Geometry: final body of the model. Coordinates: model frame, mm. Coordinates: 2 decimals unless noted, no trailing zeros. Loops run counter-clockwise (first coordinate to the right, second up) from the corner with the lowest first, then second, coordinate; pieces in that order, holes last. Notation, with made-up numbers: (-33.75, 0.5) - (-9.75, 0.5) arc R27 cw to (-9.75, 32.5) - close; hole circle Ø7 at (-10.75, 64.5). An arc over 180 degrees is marked (long way). Return JSON: item names as keys, results as strings.
from build123d import *

# Parameters (mm, degrees)
F0_W     = 130
F0_H     = 16
F1_DEPTH = 3
F2_R     = 2.575
F3_DEPTH = 3.001
F4_SIZE  = 0.2


with BuildPart() as f1:
    # F0 (on Top) → F1 (new body)
    with BuildSketch(Plane.XY):
        Rectangle(F0_W, F0_H)
    extrude(amount=F1_DEPTH)

    # F2 (on face) → F3 (cut, through all)
    with BuildSketch(Plane.XY.offset(3)):
        Circle(F2_R)
    extrude(amount=-F3_DEPTH, mode=Mode.SUBTRACT)

    # F4
    f4_edges = [f1.edges().sort_by_distance(p)[0] for p in [
        (-2.575, 0, 3),
        (-2.575, 0, 0),
    ]]
    chamfer(f4_edges, length=F4_SIZE)


solid = f1.part
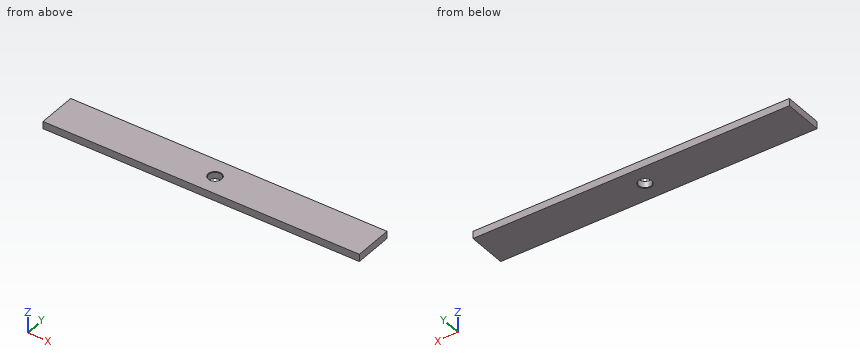
Item 1: Section query B-B, the plane x = 0. Return loops of the section in (y, z) (3 decimals), and give its area (3 significant figures).
Worked out:
{"outline": "(-8, 0) - (-2.775, 0) - (-2.575, 0.2) - (-2.575, 2.8) - (-2.775, 3) - (-8, 3) - close; (2.575, 0.2) - (2.775, 0) - (8, 0) - (8, 3) - (2.775, 3) - (2.575, 2.8) - close", "area": "32.5 mm^2"}
Item 2: Section query A-A, the plane y = 0. Return loops of the section in (x, z) (3 decimals), and give its area (3 significant figures).
Worked out:
{"outline": "(-65, 0) - (-2.775, 0) - (-2.575, 0.2) - (-2.575, 2.8) - (-2.775, 3) - (-65, 3) - close; (2.575, 0.2) - (2.775, 0) - (65, 0) - (65, 3) - (2.775, 3) - (2.575, 2.8) - close", "area": "374 mm^2"}
Item 3: Ray query, probe 1 along Y at (x, z) = (0, 2.05) (3 decimals); probe 2 along X at (y, z) = (2, 2.65); probe 3 along Y at (x, z) = (-1.5, 0.55). Return the intervals inside material, ascending. Write a range as from..to.
Worked out:
{"probe 1": "-8..-2.575, 2.575..8", "probe 2": "-65..-1.62, 1.62..65", "probe 3": "-8..-2.09, 2.09..8"}
